Autodesk Inventor part; units mm, degrees
ref_plane "YZ Plane" through (0, 0, 0) normal (1, 0, 0) x (0, 1, 0)
ref_plane "XZ Plane" through (0, 0, 0) normal (0, 1, 0) x (-1, 0, 0)
ref_plane "XY Plane" through (0, 0, 0) normal (0, 0, 1) x (1, 0, 0)
sketch "Base" plane through (0, 0, 0) normal (0, 0, 1) x (1, 0, 0)
  line L0 (-23.4822, 45.3385) -> (0, 58.896)
  line L1 (-23.4822, 13.5575) -> (-23.4822, 45.3385)
  line L2 (0, 0) -> (-23.4822, 13.5575)
  line L3 (0, 58.896) -> (0, 0)
  circle A0 centre (-11.7411, 38.3467) radius 3.175
  circle A1 centre (-11.7411, 20.5493) radius 3.175
  line L4 (-11.7411, 38.3467) -> (-11.7411, 20.5493) construction
  line L5 (-11.7411, 29.448) -> (-23.4822, 29.448) construction
  line L6 (-20.2078, 47.229) -> (-20.2078, 11.667)
  dimension "d0" = 58.896
  dimension "d1" = 27.1149
  dimension "d2" = 60
  dimension "d3" = 60
  dimension "d4" = 31.7811
  dimension "d5" = 6.35
  dimension "d6" = 17.7974
  dimension "d7" = 11.7411
  dimension "d8" = 11.7411
  dimension "d9" = 8.4667
extrude "Plate1" add sketch "Base" along normal blind 5.08 contours L0 L3 L2 L6
sketch "Sketch2" plane through (-24.9814, 47.229, -3.3425) normal (-0.9396926, 0, 0.3420201) x (0, -1, 0)
  line L0 (35.562, 0) -> (0, 0)
  line L1 (0, 0) -> (0, -24.6359)
  line L2 (0, -24.6359) -> (35.562, -24.6359)
  line L3 (35.562, -24.6359) -> (35.562, 0)
edge flange "ShockFlangeFeature" height 31.75 angle 70 thickness 5.08 bend radius 5.08 thickness toward (-0.9396926, 0, 0.3420201) relief tear relief width 5.08 relief depth 2.54 edges at (-20.2078, 29.448, 0) wall of the first edge with corners at (-24.9814, 11.667, -3.3425) (-24.9814, 47.229, -3.3425) (-33.4074, 47.229, -26.4927) (-33.4074, 11.667, -26.4927)
bend "Bend1"
corner "Corner1"
sketch "ShockFlangeDraft" plane through (-33.4074, 11.667, -26.4927) normal (0.9396926, 0, -0.3420201) x (-0.3420201, 0, -0.9396926)
  line L0 (-24.6359, 35.562) -> (-24.6359, 0)
  line L1 (0, 0) -> (-24.6359, 0)
  line L2 (0, 0) -> (0, 35.562)
  line L3 (0, 35.562) -> (-24.6359, 35.562)
  line L4 (-24.2986, 35.562) -> (0, 24.2098)
  line L5 (-24.6359, 0) -> (0, 11.5098)
  line L6 (0, 17.781) -> (-24.6359, 17.781) construction
  line L7 (-24.6359, 35.562) -> (-24.6359, 0)
  point P0 (-36.321, -11.667)
  dimension "d34" = 64.958
  dimension "d35" = 64.958
  dimension "d36" = 12.7
extrude "ShockFlangeDraftFeature" cut sketch "ShockFlangeDraft" against normal blind 25.4 contours L5 L2 L1 | L3 L2 L4
fillet "FilletsFeature" radius 6.35 6 edges at (-35.7942, 35.8768, -25.624) (0, 58.896, 2.54) (0, 0, 2.54) (-27.4836, 47.229, -2.7907) (-35.7942, 23.1768, -25.624) (-27.3682, 11.667, -2.4738)
sketch "ShockMountHole" plane through (-29.755, 11.667, -1.6051) normal (-0.9396926, 0, 0.3420201) x (0.3420201, 0, 0.9396926)
  circle A0 centre (-14.6604, 17.8598) radius 9.9755 construction
  line L0 (-24.6359, 15.5519) -> (-24.6359, 20.1677)
  line L1 (-20.9737, 25.9208) -> (-1.6149, 34.9651)
  line L2 (-1.2776, 0.5969) -> (-20.9737, 9.7989)
  circle A1 centre (-14.6604, 17.8598) radius 3.175
  point P0 (-0.1927, 28.9261)
  dimension "d37" = 6.35
hole "ShockMountHoleFeature" at (-34.7692, 29.5268, -15.3813) direction (0.9396926, 0, -0.3420201) diameter 6.35 end through all
equation "\"d35\" = d34"
equation "\"d32\" = Thickness"
equation "\"d10\" = Thickness"
equation "\"d11\" = BendReliefWidth"
equation "\"d12\" = BendReliefDepth"
equation "\"d13\" = MinimumRemnant"
equation "\"d14\" = TransitionRadius"
equation "\"d17\" = BendRadius"
equation "\"d18\" = CornerReliefSize"
equation "\"d19\" = GapSize"
equation "\"d20\" = JacobiRadiusSize"
equation "\"BendRadius\" = Thickness"
equation "\"BendReliefWidth\" = Thickness"
equation "\"BendReliefDepth\" = 0.5 * Thickness"
equation "\"CornerReliefSize\" = 4 * Thickness"
equation "\"MinimumRemnant\" = 2 * Thickness"
equation "\"TransitionRadius\" = BendRadius"
equation "\"JacobiRadiusSize\" = BendRadius"
equation "\"GapSize\" = Thickness"
properties part number "ChestPelvisConnector"
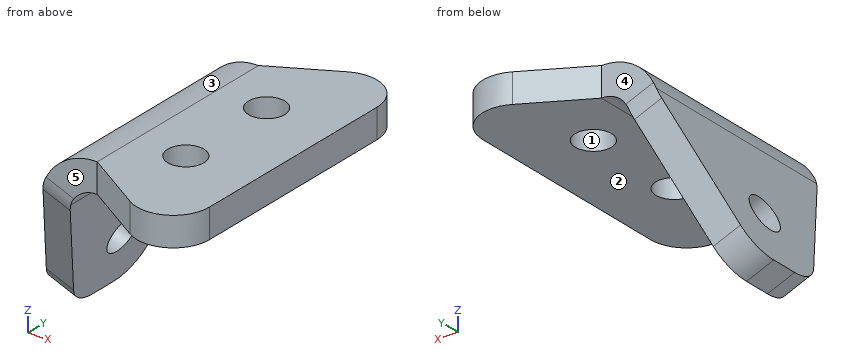
Here's how the part is built. I have some questions about the finished solid (model axes, mm). Face numbers are marked on the shaded views. A direction names the side the tool comes from. Coordinates: 2 decimals unless noted, no trailing zeros. Order: outer loops, then holes, each group sorted by start corner. A loop starts at its lowest first (then second) coordinate and runs counter-clockwise, first axis right, second up. Notation, with made-up numbers: (-6, 65.5) - (22, 65.5) arc R12 cw to (22, 86.5) - close; hole circle Ø7 at (10.25, 43.25). An arc over 180 degrees is marked (long way). One line per question, with ' | ' between items. Start each with the question number.
1. Which directions (+Z, -Z, +X, -X, +Y, -Y) give clear straight access to the entire face, cutting with the end or side of a thin tool? Please do the marked faces 1, 2, 3, 4 and 5.
2. If we section it at C-C (x = -11): Write out the boundary of the cut face in (y, z), and give its area (3 significant figures).
3. I'm going to push flat-ended pins straight in: pin 1 Ø6 at (x, y) = (-5.5, 25) entering from -Z; pin 2 Ø1.5 at (x, y) = (-9, 21.5) entering from +Z; pin 3 Ø5 at (x, y) = (-11.74, 20.55) entering from +Z; pin 4 Ø8 at (x, z) = (-26, -3.5) entering from -Y. Where does each tip first touch, or does it pass through?
4. If we section it at D-D (y = 14.5): Write out the boundary of the cut face in (x, z), and give its area (3 significant figures).
5. If we section it at B-B (y = 40): Write out the boundary of the cut face in (x, z).
6. If we section it at A-A (z = 1): Write out the boundary of the cut face in (x, y) (3 decimals), and give its area (3 significant figures).
7. Please list where these lines run through material, in increasing order: line 1 along X through (y, z) = (22, 1.5); line 2 along Y through (x, z) = (-21, 2); line 3 along Z through (x, y) = (-7.5, 8.5). Write a range as [from, to].
Model answer:
1) face 1: +Z, -Z | face 2: -Z, +X, +Y, -Y | face 3: +Z, -X, +Y, -Y | face 4: +Z, -Z, -X, +Y | face 5: +Z, -Z, -X, -Y
2) outline: (6.35, 0) - (17.46, 0) - (17.46, 5.08) - (6.35, 5.08) - close; (23.64, 0) - (35.26, 0) - (35.26, 5.08) - (23.64, 5.08) - close; (41.43, 0) - (52.55, 0) - (52.55, 5.08) - (41.43, 5.08) - close | area: 172 mm²
3) pin 1: stops at z = 0 | pin 2: stops at z = 5.08 | pin 3: passes through | pin 4: stops at y = 11.67
4) outline: (-31.83, -7.3) - (-27.06, -9.04) - (-24.98, -3.34) arc R5.08 cw to (-20.21, 0) - (0, 0) - (0, 5.08) - (-20.21, 5.08) arc R10.16 ccw to (-29.76, -1.61) - close | area: 181 mm²
5) outline: (-35.16, -16.46) - (-30.39, -18.2) - (-24.98, -3.34) arc R5.08 cw to (-20.21, 0) - (-14.45, 0) - (-14.45, 5.08) - (-20.21, 5.08) arc R10.16 ccw to (-29.76, -1.61) - close; (-9.03, 0) - (0, 0) - (0, 5.08) - (-9.03, 5.08) - close
6) outline: (-28.348, 11.667) - (-20.208, 11.667) - (-9.525, 5.499) arc R6.35 ccw to (0, 10.999) - (0, 47.897) arc R6.35 ccw to (-9.525, 53.397) - (-20.208, 47.229) - (-28.348, 47.229) - close; hole circle Ø6.35 at (-11.741, 20.549); hole circle Ø6.35 at (-11.741, 38.347) | area: 1,130 mm²
7) line 1: x = [-27.95, -14.57], [-8.92, 0] | line 2: y = [11.67, 47.23] | line 3: z = [0, 5.08]
